Geometry check sheet. Reference: the model listing, model coordinates, mm. A direction names the side the tool comes from. Coordinates: 2 decimals unless noted, no trailing zeros. Loops run counter-clockwise (first coordinate to the right, second up) from the corner with the lowest first, then second, coordinate; pieces in that order, holes last. Notation, with made-up numbers: (4, 82.25) -> (31, 82.25) arc R31 cw to (31, 116.25) -> close; hole circle Ø3 at (-31, 7.25). An arc over 180 degrees is marked (long way). Answer as a JSON object with one key per item and string values.
from build123d import *

# Parameters (mm, degrees)
CROQUIS1_W              = 130
CROQUIS1_H              = 116
SALIENTE_EXTRUIR1_DEPTH = 39.5
CORTAR_EXTRUIR1_DEPTH   = 39.5
REDONDEO1_R             = 5


with BuildPart() as part:
    # Croquis1 → Saliente-Extruir1 (new body)
    with BuildSketch(Plane.XY):
        with Locations((10.583554643, -12.877675841)):
            Rectangle(CROQUIS1_W, CROQUIS1_H)
    extrude(amount=SALIENTE_EXTRUIR1_DEPTH)

    # Croquis2 → Cortar-Extruir1 (cut)
    with BuildSketch(Plane.XY.offset(39.5)):
        Polygon((-44.901782094, 36.331293299), (66.068891381, 36.331293299), (10.583554643, -5.790794085), align=None)
        Polygon((-44.901782094, 22.157529787), (-44.901782094, -47.912881469), (1.248356768, -12.877675841), align=None)
        Polygon((19.918752519, -12.877675841), (66.068891381, 22.157529787), (66.068891381, -47.912881469), align=None)
        Polygon((-44.901782094, -62.086644981), (10.583554643, -19.964557597), (66.068891381, -62.086644981), align=None)
    extrude(amount=-CORTAR_EXTRUIR1_DEPTH, mode=Mode.SUBTRACT)

    # Redondeo1
    redondeo1_edges = [part.edges().sort_by_distance(p)[0] for p in [
        (10.583554643, -5.790794085, 19.75),
        (-44.901782094, 36.331293299, 19.75),
        (66.068891381, 36.331293299, 19.75),
        (-44.901782094, 22.157529787, 19.75),
        (1.248356768, -12.877675841, 19.75),
        (-44.901782094, -47.912881469, 19.75),
        (66.068891381, -47.912881469, 19.75),
        (19.918752519, -12.877675841, 19.75),
        (66.068891381, 22.157529787, 19.75),
        (66.068891381, -62.086644981, 19.75),
        (-44.901782094, -62.086644981, 19.75),
        (10.583554643, -19.964557597, 19.75),
        (-54.416445357, 45.122324159, 19.75),
        (75.583554643, 45.122324159, 19.75),
        (75.583554643, -70.877675841, 19.75),
        (-54.416445357, -70.877675841, 19.75),
    ]]
    fillet(redondeo1_edges, radius=REDONDEO1_R)


solid = part.part
1. Mould release check, pull along Y, two halves, no side actions. Record for faces 1 (the face through (-12.47, 11.71, 20.03)), 2 (the face through (-52.99, 43.62, 20.03)), 3 (the face through (10, -12, 39.5)): released by +Y, released by -Y, zero draft, split by the parting line, or undercut.
Evaluation:
{"face 1": "undercut", "face 2": "released by +Y", "face 3": "zero draft"}
2. Section check C-C, the plane y = 24.5. Record the boundary of the cut face in (x, z).
Evaluation:
{"outline": "(-54.42, 0) -> (-29.32, 0) -> (-29.32, 39.5) -> (-54.42, 39.5) -> close; (50.48, 0) -> (75.58, 0) -> (75.58, 39.5) -> (50.48, 39.5) -> close"}
3. Section check A-A, the plane z = 5. State how many separate pieces and enclosed holes the cut face has, then the cut area to 3 significant figures.
Evaluation:
{"separate pieces": "1", "enclosed holes": "4", "area": "7,440 mm^2"}
4. Section check D-D, the plane y = -40. Record the boundary of the cut face in (x, z).
Evaluation:
{"outline": "(-54.42, 0) -> (-44.41, 0) -> (-44.41, 39.5) -> (-54.42, 39.5) -> close; (-34.48, 0) -> (-15.81, 0) -> (-15.81, 39.5) -> (-34.48, 39.5) -> close; (36.98, 0) -> (55.65, 0) -> (55.65, 39.5) -> (36.98, 39.5) -> close; (65.58, 0) -> (75.58, 0) -> (75.58, 39.5) -> (65.58, 39.5) -> close"}
5. Thickness scan on probe 1 along Y at (x, z) = (61, 10.5); probe 2 along Y at (x, z) = (7, 14); probe 3 along X at (y, z) = (-26.5, 12.5). Record the ranges inside material, lowest first. Write a range as from..to.
Evaluation:
{"probe 1": "y = -70.88..-42.84, 17.08..45.12", "probe 2": "y = -70.88..-62.09, -22.69..-3.07, 36.33..45.12", "probe 3": "x = -54.42..-44.9, -16.7..1.97, 19.19..37.86, 66.07..75.58"}
6. Section check B-B, the plane x = -8.5. Record the boundary of the cut face in (y, z), then the cut area to 3 significant figures.
Evaluation:
{"outline": "(-70.88, 0) -> (-62.09, 0) -> (-62.09, 39.5) -> (-70.88, 39.5) -> close; (-34.45, 0) -> (-20.28, 0) -> (-20.28, 39.5) -> (-34.45, 39.5) -> close; (-5.48, 0) -> (8.7, 0) -> (8.7, 39.5) -> (-5.48, 39.5) -> close; (36.33, 0) -> (45.12, 0) -> (45.12, 39.5) -> (36.33, 39.5) -> close", "area": "1,810 mm^2"}
7. Tool access check on faces 4 (the face through (74.08, -69.45, 20.03)), 5 (the face through (10.538, -4.513, 19.474)). Record the directions out of +Z, -Z, +X, -X, +Y, -Y that give a thin tool (end or side, any length) a straight path to the whole face; none if there is none.
Evaluation:
{"face 4": "+Z, -Z, +X, -Y", "face 5": "+Z, -Z"}
